Could you check a few things on this model? Use its own coordinates, in mm. A direction names the side the tool comes from. Give positions to 0.01 mm unless a question says otherwise; leave off trailing zeros. Write each loop counter-clockwise with the first axis right and the second up, starting at its lowest first coordinate (ties: lowest second). Pieces come first, ordered by that corner, then holes. Notation, with made-up numbers: M 18,79.5 L 44,79.5 A18 ccw 44,102.5 Z; hole C 80,45.25 d8. An arc over 180 degrees is marked long. Use one line per item in the form item = value.
from build123d import *


with BuildPart() as part:
    # Sketch1 → Base-Revolve (revolve)
    with BuildSketch(Plane.XY):
        with BuildLine():
            Line((-145, 35), (-145, 46.5))
            ThreePointArc((-145, 46.5), (-144.707106781, 47.207106781), (-144, 47.5))
            Line((-144, 47.5), (144, 47.5))
            ThreePointArc((144, 47.5), (144.707106781, 47.207106781), (145, 46.5))
            Line((145, 46.5), (145, 35))
            Line((145, 35), (65, 35))
            Line((65, 35), (58.296999614, 37.439692621))
            ThreePointArc((58.296999614, 37.439692621), (58.128627648, 37.484807753), (57.954979471, 37.5))
            Line((57.954979471, 37.5), (-57.954979471, 37.5))
            ThreePointArc((-57.954979471, 37.5), (-58.128627648, 37.484807753), (-58.296999614, 37.439692621))
            Line((-58.296999614, 37.439692621), (-65, 35))
            Line((-65, 35), (-145, 35))
        make_face()
    revolve(axis=Axis((-145, 0, 0), (1, 0, 0)))

    # Sketch5 → 2.5 x 30 gr reifning (revolve, cut)
    with BuildSketch(Plane.XY):
        Polygon((145, 35.866025404), (143.5, 35), (145, 35), align=None)
        Polygon((-145, 35), (-145, 35.866025404), (-143.5, 35), align=None)
    revolve(axis=Axis((0, 0, 0), (1, 0, 0)), mode=Mode.SUBTRACT)


solid = part.part
1) Thinking about a two-plate mould opening in X: for faces 3 (the flat face through (-145, -24, -27)), 4 (the conical face through (-64.67, 33.5, 10.55)), 5 (the conical face through (64.58, 33.53, 10.56)), 6 (the cylindrical face through (2.02, -10.3, -46.37)), which applies, released by +X, released by -X, zero draft, split by the parting line, or undercut?
Checked values:
face_3 = released by -X
face_4 = undercut
face_5 = undercut
face_6 = zero draft
2) I want a section at D-D, the plane x = -12.5. Please give me the cut outline in (y, z).
Checked values:
outline = C 0,0 d95; hole C 0,0 d75
3) For pin 1 Ø6 at (x, z) = (-86, 6.5) entering from -Y; pin 2 Ø6 at (x, z) = (67, -31) entering from -Y; pin 3 Ø1 at (x, z) = (38.5, -19) entering from +Y, each with a flat end and sliding along its axis, tell me the tip position at first contact or that it passes through.
Checked values:
pin_1 = -47.37
pin_2 = -38.37
pin_3 = 43.75
4) If I drill on L1, parallel to Z at x = -10, y = 0; L2, parallel to Y at x = -110, z = -5; L3, parallel to Y at x = 62, z = 12, over which ranges is the centre line in solid material (lowest first)?
Checked values:
L1 = -47.5 to -37.5, 37.5 to 47.5
L2 = -47.24 to -34.64, 34.64 to 47.24
L3 = -45.96 to -34.04, 34.04 to 45.96
5) For faces 1 (the cylindrical face through (-105, -28, -21)), 2 (the cylindrical face through (-0.81, -4.88, 37.18)), which set-ups out of +Z, -Z, +X, -X, +Y, -Y let a thin tool reach every point of the face, with its end or its side?
Checked values:
face_1 = +X, -X
face_2 = none
6) I want a section at A-A, the plane y = 0. Please give me the cut outline in (x, z), plus the area to 3 significant figures.
Checked values:
outline = M -145,-46.5 A1 ccw -144,-47.5 L 144,-47.5 A1 ccw 145,-46.5 L 145,-35.87 L 143.5,-35 L 65,-35 L 58.3,-37.44 A1 cw 57.95,-37.5 L -57.95,-37.5 A1 cw -58.3,-37.44 L -65,-35 L -143.5,-35 L -145,-35.87 Z; M -145,35.87 L -143.5,35 L -65,35 L -58.3,37.44 A1 cw -57.95,37.5 L 57.95,37.5 A1 cw 58.3,37.44 L 65,35 L 143.5,35 L 145,35.87 L 145,46.5 A1 ccw 144,47.5 L -144,47.5 A1 ccw -145,46.5 Z
area = 6,630 mm2
7) I want a section at C-C, the plane x = -93.5. Please give me the cut outline in (y, z), plus the area to 3 significant figures.
Checked values:
outline = C 0,0 d95; hole C 0,0 d70
area = 3,240 mm2
